Verification items for the finished model (mm, model axes). Face numbers are marked on the shaded views. A direction names the side the tool comes from. Give positions to 0.01 mm unless a question says otherwise; leave off trailing zeros. Write each loop counter-clockwise with the first axis right and the second up, starting at its lowest first coordinate (ties: lowest second). Pieces come first, ordered by that corner, then holes. Notation, with made-up numbers: (-18.75, -18.75) - (15.25, -18.75) arc R25 cw to (15.25, 12.25) - close; hole circle Ø1 at (22.25, -39.75). An arc over 180 degrees is marked (long way). Answer as a JSON object with one key per item and string values. Group by question number.
Item 1: Scan lines: line 1 along Z through (x, y) = (13.5, 1.75); line 2 along Z through (x, y) = (7, 0.25); line 3 along Y through (x, z) = (17, -6.25). Record each from-to range of solid material in increasing order. Write a range as [from, to].
Item 2: Sectioned sample at C-C, the plane z = -1.5. Record the boundary of the cut face in (x, y).
Item 3: Draft check along Z on the marked faces 1, 2 and 3. Enter one of: +Z half, -Z half, draft (parallel to the pull), parting line (faces both ways), or undercut.
Item 4: Tool access check on the marked faces 4, 5 and 6. Record the directions out of +Z, -Z, +X, -X, +Y, -Y that give a thin tool (end or side, any length) a straight path to the whole face; none if there is none.
Item 5: Sectioned sample at A-A, the plane x = 10.25. Record the boundary of the cut face in (y, z), and give its area (3 significant figures).
Item 6: Sectioned sample at B-B, the plane z = -21. Record the boundary of the cut face in (x, y) (3 decimals), and give its area (3 significant figures).
Item 7: Sectioned sample at D-D, the plane z = -7. Record the boundary of the cut face in (x, y), and give its area (3 significant figures).
Item 8: Go/stop test with flat-tipped pins: pin 1 (2.5 mm diameter, centred on y = -1, z = -2.5, fed in from +X); pin 2 (0.6 mm diameter, centred on y = 1, z = -20, fed in from +X); pin 3 (1 mm diameter, centred on y = -3, z = -20.5, fed in from +X); pin 4 (1.3 mm diameter, centred on x = 1, y = -2.5, fed in from +Z). Record where each tip stops, or that it passes through.
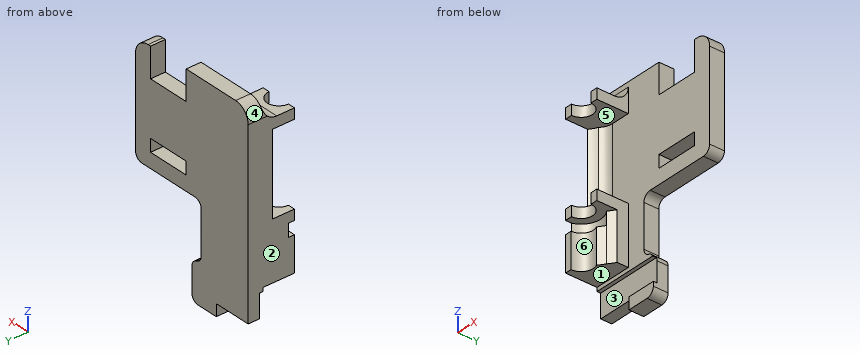
```python
from build123d import *

# Parameters (mm, degrees)
SKETCH1_W               = 18
SKETCH1_H               = 28
BOSS_EXTRUDE1_DEPTH     = 2
SKETCH2_W               = 5
SKETCH2_H               = 1.4
BOSS_EXTRUDE2_DEPTH     = 4.25
CUT_EXTRUDE1_DEPTH      = 34.556854739
CUT_EXTRUDE1_DEPTH_BACK = 34.556854739
SKETCH4_R               = 1.55
FILLET1_R               = 2
SKETCH5_W               = 5.7
SKETCH5_H               = 1.7
SKETCH5_H_2             = 4
SKETCH5_W_2             = 5.1
SKETCH5_H_3             = 1.6
CUT_EXTRUDE2_DEPTH      = 2
CUT_EXTRUDE3_DEPTH      = 34.868311148
CUT_EXTRUDE3_DEPTH_BACK = 34.868311148
FILLET2_R               = 2
SKETCH8_W               = 5.25
SKETCH8_H               = 2
BOSS_EXTRUDE3_DEPTH     = 1.5
FILLET3_R               = 1
FILLET4_R               = 1
SKETCH7_W               = 3.15
SKETCH7_H               = 0.5
CUT_EXTRUDE4_DEPTH      = 34.556854876
BOSS_EXTRUDE4_REACH     = 32.379
BOSS_EXTRUDE6_DEPTH     = 6.45
BOSS_EXTRUDE7_START     = -4.7
BOSS_EXTRUDE7_DEPTH     = 4.7
FILLET7_R               = 2
FILLET8_R               = 1.85


with BuildPart() as part:
    # Sketch1 → Boss-Extrude1 (new body)
    with BuildSketch(Plane(origin=(0, 0, 0), x_dir=(1, 0, 0), z_dir=(0, 1, 0))):
        with Locations((9, 14)):
            Rectangle(SKETCH1_W, SKETCH1_H)
    extrude(amount=BOSS_EXTRUDE1_DEPTH)

    # Sketch2 → Boss-Extrude2 (add)
    with BuildSketch(Plane.XZ):
        with Locations((2.5, -3.2)):
            Rectangle(SKETCH2_W, SKETCH2_H)
        with Locations((2.5, -15.6)):
            Rectangle(SKETCH2_W, SKETCH2_H)
    extrude(amount=BOSS_EXTRUDE2_DEPTH)

    # Sketch4 → Cut-Extrude1 (cut, two sides: drawn at the far end of the back side and taken through both)
    with BuildSketch(Plane.XY.offset(-CUT_EXTRUDE1_DEPTH_BACK)):
        with Locations((2.5, -4.25)):
            Circle(SKETCH4_R)
    extrude(amount=CUT_EXTRUDE1_DEPTH + CUT_EXTRUDE1_DEPTH_BACK, mode=Mode.SUBTRACT)

    # Fillet1
    fillet1_edges = [part.edges().sort_by_distance(p)[0] for p in [
        (0, 1, 0),
    ]]
    fillet(fillet1_edges, radius=FILLET1_R)

    # Sketch5 → Cut-Extrude2 (cut)
    with BuildSketch(Plane(origin=(0, 2, 0), x_dir=(1, 0, 0), z_dir=(0, 1, 0))):
        with Locations((12.75, 12.15)):
            Rectangle(SKETCH5_W, SKETCH5_H)
        with Locations((12.75, 2)):
            Rectangle(SKETCH5_W, SKETCH5_H_2)
        with Locations((2.55, 27.2)):
            Rectangle(SKETCH5_W_2, SKETCH5_H_3)
    extrude(amount=-CUT_EXTRUDE2_DEPTH, mode=Mode.SUBTRACT)

    # Sketch6 → Cut-Extrude3 (cut, two sides: drawn at the far end of the back side and taken through both)
    with BuildSketch(Plane(origin=(0, 2, 0), x_dir=(1, 0, 0), z_dir=(0, 1, 0)).offset(-CUT_EXTRUDE3_DEPTH_BACK)):
        with BuildLine():
            Line((18, 14), (20.5, 14))
            Line((20.5, 14), (20.5, 30.5))
            Line((20.5, 30.5), (7.5, 30.5))
            Line((7.5, 30.5), (7.5, 28))
            Line((7.5, 28), (7.5, 16))
            ThreePointArc((7.5, 16), (7.792893219, 15.292893219), (8.5, 15))
            Line((8.5, 15), (17, 15))
            ThreePointArc((17, 15), (17.707106781, 14.707106781), (18, 14))
        make_face()
    extrude(amount=CUT_EXTRUDE3_DEPTH + CUT_EXTRUDE3_DEPTH_BACK, mode=Mode.SUBTRACT)

    # Fillet2
    fillet2_edges = [part.edges().sort_by_distance(p)[0] for p in [
        (18, 1, 0),
    ]]
    fillet(fillet2_edges, radius=FILLET2_R)

    # Sketch8 → Boss-Extrude3 (add)
    with BuildSketch(Plane(origin=(7.5, 0, 0), x_dir=(0, 0, -1), z_dir=(1, 0, 0))):
        with Locations((25.375, 1)):
            Rectangle(SKETCH8_W, SKETCH8_H)
    extrude(amount=BOSS_EXTRUDE3_DEPTH)

    # Fillet3
    fillet3_edges = [part.edges().sort_by_distance(p)[0] for p in [
        (7.5, 1, -22.75),
        (9, 1, -28),
    ]]
    fillet(fillet3_edges, radius=FILLET3_R)

    # Fillet4
    fillet4_edges = [part.edges().sort_by_distance(p)[0] for p in [
        (9, 1, -22.75),
    ]]
    fillet(fillet4_edges, radius=FILLET4_R)

    # Sketch7 → Cut-Extrude4 (cut, through all)
    with BuildSketch(Plane.ZY):
        with Locations((-24.825, 0.25)):
            Rectangle(SKETCH7_W, SKETCH7_H)
    extrude(amount=-CUT_EXTRUDE4_DEPTH, mode=Mode.SUBTRACT)

    # Sketch9 → Boss-Extrude4 (add, up to next)
    with BuildSketch(Plane(origin=(0, 0, -3.9), x_dir=(-1, 0, 0), z_dir=(0, 0, -1)), mode=Mode.PRIVATE) as boss_extrude4_sk1:
        with BuildLine():
            Line((0, 0), (-1, 0))
            Line((-1, 0), (-1, -0.65))
            ThreePointArc((-1, -0.65), (-0.477127448, -0.915635497), (0, -1.256674091))
            Line((0, -1.256674091), (0, 0))
        make_face()
    boss_extrude4_tool1 = extrude(boss_extrude4_sk1.sketch, amount=BOSS_EXTRUDE4_REACH, mode=Mode.PRIVATE) - part.part
    add(boss_extrude4_tool1.solids().sort_by_distance((0.445326, -0.476066, -3.9))[0])

    # Sketch10 → Boss-Extrude6 (add)
    with BuildSketch(Plane(origin=(0, 0, -16.3), x_dir=(-1, 0, 0), z_dir=(0, 0, -1))):
        with BuildLine():
            Line((-5, -1.5), (-4.075, -2.15))
            ThreePointArc((-4.075, -2.15), (-1.702408348, -1.749105649), (0, -3.44960947))
            Line((0, -3.44960947), (0, 0))
            Line((0, 0), (-5, 0))
            Line((-5, 0), (-5, -1.5))
        make_face()
    extrude(amount=BOSS_EXTRUDE6_DEPTH)

    # Sketch11 → Boss-Extrude7 (add)
    with BuildSketch(Plane(origin=(0, 0, -22.75), x_dir=(-1, 0, 0), z_dir=(0, 0, -1)).offset(BOSS_EXTRUDE7_START)):
        with BuildLine():
            Line((-4.075, -2.15), (-3.184119692, -2.776024))
            ThreePointArc((-3.184119692, -2.776024), (-1.625662965, -2.880270191), (-0.875, -4.25))
            Line((-0.875, -4.25), (0, -4.25))
            Line((0, -4.25), (0, -3.44960947))
            ThreePointArc((0, -3.44960947), (-1.702408348, -1.749105649), (-4.075, -2.15))
        make_face()
    extrude(amount=BOSS_EXTRUDE7_DEPTH)

    # Fillet7
    # the kernel refuses this fillet: 2 mm, written as the material it adds along each edge
    with BuildSketch(Plane(origin=(1, 0, -3.9), x_dir=(1, 0, 0), z_dir=(0, 0, -1))) as fillet7_piece_1:
        with BuildLine():
            CenterArc((1.475635456, 2), FILLET7_R, 222.454150204, 47.545849796)
            Line((0, 0.65), (0, 0))
            Line((0, 0), (1.475635456, 0))
        make_face()
    extrude(amount=14.689088641)

    # Fillet8
    fillet8_edges = [part.edges().sort_by_distance(p)[0] for p in [
        (2.5, 0, -2.5),
    ]]
    fillet(fillet8_edges, radius=FILLET8_R)


solid = part.part
```
Geometry check:
{
 "1": {"line 1": "[-15, -13], [-11.3, -4]", "line 2": "[-28, -26.4], [-23.25, 0]", "line 3": "[0, 2]"},
 "2": {"outline": "(0.06, -0.21) - (5, -0.21) - (5, 0) - (9.9, 0) - (9.9, 2) - (0.06, 2) - close; (15.6, 0) - (17.94, 0) - (17.94, 2) - (15.6, 2) - close"},
 "3": {"face 1": "-Z half", "face 2": "draft", "face 3": "undercut"},
 "4": {"face 4": "+Z, -X, +Y, -Y", "face 5": "+X, -Y", "face 6": "-Z, -Y"},
 "5": {"outline": "(0, -15) - (2, -15) - (2, -13) - (0, -13) - close; (0, -11.3) - (2, -11.3) - (2, -4) - (0, -4) - close", "area": "18.6 mm^2"},
 "6": {"outline": "(0, -4.25) - (0.875, -4.25) arc R1.625 cw to (3.184, -2.776) - (5, -1.5) - (5, 0) - (7.5, 0) - (7.5, 2) - (0, 2) - close", "area": "29.3 mm^2"},
 "7": {"outline": "(0, -1.26) arc R3.9 cw to (1, -0.65) arc R2 cw to (2.48, 0) - (18, 0) - (18, 2) - (0, 2) - close", "area": "37.2 mm^2"},
 "8": {"pin 1": "x = 18", "pin 2": "x = 7.5", "pin 3": "x = 3.58", "pin 4": "z = -2.5"}
}
